```python
from build123d import *

# Parameters (mm, degrees)
SKETCH_W        = 104
SKETCH_H        = 34
PAD_DEPTH       = 33
SKETCH001_W     = 96
SKETCH001_H     = 30
POCKET_DEPTH    = 33.001
POCKET001_DEPTH = 104.001
POCKET002_DEPTH = 2
POCKET003_DEPTH = 2


with BuildPart() as part:
    # Sketch → Pad (new body)
    with BuildSketch(Plane.XY):
        with Locations((0, 17)):
            Rectangle(SKETCH_W, SKETCH_H)
    extrude(amount=PAD_DEPTH)

    # Sketch001 (on Face6 of Pad) → Pocket (cut, through all)
    with BuildSketch(Plane.XY.offset(33)):
        with Locations((0, 15)):
            Rectangle(SKETCH001_W, SKETCH001_H)
    extrude(amount=-POCKET_DEPTH, mode=Mode.SUBTRACT)

    # Sketch002 (on Face7 of Pocket) → Pocket001 (cut, through all)
    with BuildSketch(Plane.YZ.offset(52)):
        with BuildLine():
            ThreePointArc((11.55, 28), (10, 29.55), (8.45, 28))
            Line((8.45, 28), (8.45, 25))
            ThreePointArc((8.45, 25), (10, 23.45), (11.55, 25))
            Line((11.55, 25), (11.55, 28))
        make_face()
        with BuildLine():
            ThreePointArc((11.55, 12), (10, 13.55), (8.45, 12))
            Line((8.45, 12), (8.45, 9))
            ThreePointArc((8.45, 9), (10, 7.45), (11.55, 9))
            Line((11.55, 9), (11.55, 12))
        make_face()
    extrude(amount=-POCKET001_DEPTH, mode=Mode.SUBTRACT)

    # Sketch003 (on Face7 of Pocket001) → Pocket002 (cut)
    with BuildSketch(Plane.YZ.offset(52)):
        with BuildLine():
            ThreePointArc((13.05, 28), (10, 31.05), (6.95, 28))
            Line((6.95, 28), (6.95, 25))
            ThreePointArc((6.95, 25), (10, 21.95), (13.05, 25))
            Line((13.05, 25), (13.05, 28))
        make_face()
        with BuildLine():
            ThreePointArc((13.05, 12), (10, 15.05), (6.95, 12))
            Line((6.95, 12), (6.95, 9))
            ThreePointArc((6.95, 9), (10, 5.95), (13.05, 9))
            Line((13.05, 9), (13.05, 12))
        make_face()
    extrude(amount=-POCKET002_DEPTH, mode=Mode.SUBTRACT)

    # Sketch004 (on Face5 of Pocket002) → Pocket003 (cut)
    with BuildSketch(Plane(origin=(-52, 0, 0), x_dir=(0, -1, 0), z_dir=(-1, 0, 0))):
        with BuildLine():
            ThreePointArc((-6.95, 28), (-10, 31.05), (-13.05, 28))
            Line((-13.05, 28), (-13.05, 25))
            ThreePointArc((-13.05, 25), (-10, 21.95), (-6.95, 25))
            Line((-6.95, 25), (-6.95, 28))
        make_face()
        with BuildLine():
            ThreePointArc((-6.95, 12), (-10, 15.05), (-13.05, 12))
            Line((-13.05, 12), (-13.05, 9))
            ThreePointArc((-13.05, 9), (-10, 5.95), (-6.95, 9))
            Line((-6.95, 9), (-6.95, 12))
        make_face()
    extrude(amount=-POCKET003_DEPTH, mode=Mode.SUBTRACT)


solid = part.part
```
Could you check a few things on this model? Use its own coordinates, in mm. A direction names the side the tool comes from. Coordinates: 2 decimals unless noted, no trailing zeros. Write each loop counter-clockwise with the first axis right and the second up, starting at its lowest first coordinate (ties: lowest second). Pieces come first, ordered by that corner, then holes. Notation, with made-up numbers: (-16.5, 8) -> (0.5, 8) arc R37 cw to (0.5, 44) -> close; hole circle Ø7 at (-12.75, 45.25). An arc over 180 degrees is marked (long way). Write item = value, one per line. Start each with the question number.
(1) Which directions (+Z, -Z, +X, -X, +Y, -Y) give clear straight access to the entire face, cutting with the end or side of a thin tool? Please do faces 1 (the face through (-50, 8, 11)), 2 (the face through (52, 17, 16)), 3 (the face through (-49, 8.45, 11)), 4 (the face through (51.01, 10.07, 15.05)).
(2) I want a section at C-C (y = 10). Give the number of separate pieces and of enclosed holes in the cut face, plus the area to 3 significant figures.
(3) I need wall thicknesses on line 1 (X direction, y = 12, z = 4.5); line 2 (Y direction, x = -35, z = 25). Which ranges of each line are inside material? Lowest first, please. Write a range as [from, to].
(4) We'd pull the mould along Y, two halves only. Please class faces 5 (the face through (-1, 30, 17)), 6 (the face through (-1, 34, 16)), 7 (the face through (-48, 15, 17)), 8 (the face through (-49, 11.55, 10)): released by +Y, released by -Y, zero draft, split by the parting line, or undercut.
(5) I want a section at A-A (z = 10). Please give me the cut outline in (x, y), plus the area to 3 significant figures.
(6) I want a section at D-D (x = 23.5). Please give me the cut outline in (y, z).
(7) Will this pin go through, and if not, where does the flat tip stop? pin 1 (5 mm diameter, centred on x = 12.5, z = 22, fed in from -Y).
(8) I want a section at B-B (y = 18.5). Please give me the cut outline in (x, z), plus the area to 3 significant figures.
Result set:
q1.face_1 = -X
q1.face_2 = +Z, -Z, +X, +Y, -Y
q1.face_3 = +X, -X
q1.face_4 = +X
q2.separate_pieces = 6
q2.enclosed_holes = 0
q2.area = 142 mm2
q3.line_1 = [-52, -48], [48, 52]
q3.line_2 = [30, 34]
q4.face_5 = released by -Y
q4.face_6 = released by +Y
q4.face_7 = zero draft
q4.face_8 = undercut
q5.outline = (-52, 0) -> (-48, 0) -> (-48, 8.45) -> (-50, 8.45) -> (-50, 6.95) -> (-52, 6.95) -> close; (-52, 13.05) -> (-50, 13.05) -> (-50, 11.55) -> (-48, 11.55) -> (-48, 30) -> (48, 30) -> (48, 11.55) -> (50, 11.55) -> (50, 13.05) -> (52, 13.05) -> (52, 34) -> (-52, 34) -> close; (48, 0) -> (52, 0) -> (52, 6.95) -> (50, 6.95) -> (50, 8.45) -> (48, 8.45) -> close
q5.area = 619 mm2
q6.outline = (30, 0) -> (34, 0) -> (34, 33) -> (30, 33) -> close
q7.pin_1 = 30
q8.outline = (-52, 0) -> (-48, 0) -> (-48, 33) -> (-52, 33) -> close; (48, 0) -> (52, 0) -> (52, 33) -> (48, 33) -> close
q8.area = 264 mm2
